Drawing for the job (mm, zero at the part's lowest x, y, z). A direction names the side the tool comes from. Round coordinates to 2 decimals unless told otherwise and drop trailing zeros. Write each loop counter-clockwise with the first axis right and the second up, starting at its lowest first coordinate (ties: lowest second). Pieces come first, ordered by that corner, then holes.
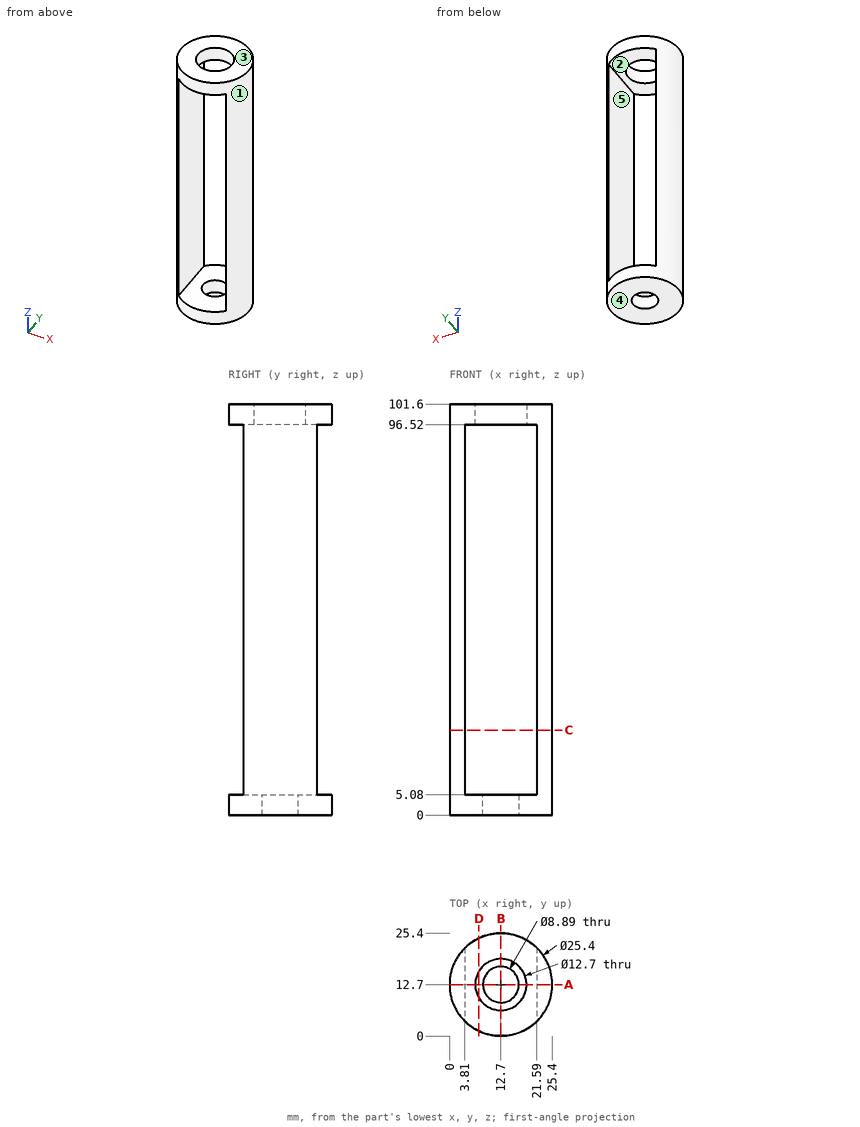
Q1. Saw through at C-C, the plane z = 21. Write the cut outline in (x, y).
Q2. Saw through at A-A, the plane y = 12.7. Write the cut outline in (x, z) (3 decimals), and give its area (3 significant figures).
Q3. Saw through at B-B, the plane x = 12.7. Write the cut outline in (y, z) (3 decimals), and give its area (3 significant figures).
Q4. Two-plate mould, pull along Z, no slides. Class the marked faces 3, 4 and 5: released by +Z, released by -Z, zero draft, split by the parting line, or undercut.
Q5. Drop flat-ended pins along their axis: P1, Ø3, axis at y = 21.5, z = 48.5, coming from the -X side; P2, Ø2, axis at y = 9, z = 67.5, coming from the +X side; P3, Ø1, axis at x = 22.5, z = 84.5, coming from the -Y side. Give the stop position or say it passes through.
Q6. Saw through at D-D, the plane x = 7.25. Write the cut outline in (y, z).
Q7. Wall check: line 1 (Z direction, x = 6.5, y = 7); line 2 (Y direction, x = 12.7, z = 1.85) (3 decimals); line 3 (Y direction, x = 12.7, z = 99.15). Give the ranges that are in metal, low to high.
Q8. Tool access for the marked faces 1 and 2: list every direction of +Z, -Z, +X, -X, +Y, -Y with a clear straight run to the whole face (end or side of a thin tool).
Computed:
1. outline: (3.81, 3.63) - (3.81, 21.77) arc R12.7 ccw to start; (21.59, 3.63) arc R12.7 ccw to (21.59, 21.77) - close
2. outline: (0, 0) - (8.255, 0) - (8.255, 5.08) - (3.81, 5.08) - (3.81, 96.52) - (6.35, 96.52) - (6.35, 101.6) - (0, 101.6) - close; (17.145, 0) - (25.4, 0) - (25.4, 101.6) - (19.05, 101.6) - (19.05, 96.52) - (21.59, 96.52) - (21.59, 5.08) - (17.145, 5.08) - close
2. area: 845 mm2
3. outline: (0, 0) - (8.255, 0) - (8.255, 5.08) - (0, 5.08) - close; (0, 96.52) - (6.35, 96.52) - (6.35, 101.6) - (0, 101.6) - close; (17.145, 0) - (25.4, 0) - (25.4, 5.08) - (17.145, 5.08) - close; (19.05, 96.52) - (25.4, 96.52) - (25.4, 101.6) - (19.05, 101.6) - close
3. area: 148 mm2
4. face 3: released by +Z
4. face 4: released by -Z
4. face 5: undercut
5. P1: stops at x = 2.31
5. P2: stops at x = 25.11
5. P3: stops at y = 4.05
6. outline: (1.23, 0) - (24.17, 0) - (24.17, 5.08) - (1.23, 5.08) - close; (1.23, 96.52) - (9.44, 96.52) - (9.44, 101.6) - (1.23, 101.6) - close; (15.96, 96.52) - (24.17, 96.52) - (24.17, 101.6) - (15.96, 101.6) - close
7. line 1: z = 0 to 5.08, 96.52 to 101.6
7. line 2: y = 0 to 8.255, 17.145 to 25.4
7. line 3: y = 0 to 6.35, 19.05 to 25.4
8. face 1: +Z, -Z
8. face 2: +Y, -Y
